CAD build for the part. Positions are in the model's coordinates, mm. A direction names the side the tool comes from. Give positions to 0.01 mm unless a question says otherwise; leave off trailing zeros. Write each loop counter-clockwise with the first axis right and the second up, starting at its lowest first coordinate (ties: lowest second). Pieces come first, ordered by that corner, then holes. Notation, with made-up numbers: (42, 70.25) - (92, 70.25) arc R30 ccw to (92, 105.25) - close; hole circle Ø11 at (2, -8.5). An arc over 180 degrees is marked (long way). Answer as a JSON object with one key per item and string values.
from build123d import *

# Parameters (mm, degrees)
CUT_EXTRUDE1_START = -4.25
SKETCH2_R          = 11.5
SKETCH2_R_2        = 11
CUT_EXTRUDE1_DEPTH = 1
CUT_EXTRUDE2_START = -12.75
SKETCH2_2_R        = 11.5
SKETCH2_2_R_2      = 11
CUT_EXTRUDE2_DEPTH = 1
SCALE1_SCALE       = 1.013


with BuildPart() as part:
    # Sketch1 → Revolve1 (revolve)
    with BuildSketch(Plane(origin=(0, 0, 0), x_dir=(0, 0, -1), z_dir=(1, 0, 0)), mode=Mode.PRIVATE) as revolve1_sk:
        with BuildLine():
            Line((-7, 11), (7, 11))
            Line((7, 11), (8, 12))
            Line((8, 12), (8, 19))
            ThreePointArc((8, 19), (7.707106781, 19.707106781), (7, 20))
            Line((7, 20), (6.5, 20))
            ThreePointArc((6.5, 20), (0, 13.5), (-6.5, 20))
            Line((-6.5, 20), (-7, 20))
            ThreePointArc((-7, 20), (-7.707106781, 19.707106781), (-8, 19))
            Line((-8, 19), (-8, 12))
            Line((-8, 12), (-7, 11))
        make_face()
    revolve(revolve1_sk.sketch.rotate(Axis((0, 0, 0), (0, 0, -1)), 90), axis=Axis((0, 0, 0), (0, 0, -1)))

    # Sketch2 → Cut-Extrude1 (cut)
    with BuildSketch(Plane.XY.offset(8).offset(CUT_EXTRUDE1_START)):
        Circle(SKETCH2_R)
        Circle(SKETCH2_R_2, mode=Mode.SUBTRACT)
    extrude(amount=CUT_EXTRUDE1_DEPTH, mode=Mode.SUBTRACT)

    # Sketch2_2 → Cut-Extrude2 (cut)
    with BuildSketch(Plane.XY.offset(8).offset(CUT_EXTRUDE2_START)):
        Circle(SKETCH2_2_R)
        Circle(SKETCH2_2_R_2, mode=Mode.SUBTRACT)
    extrude(amount=CUT_EXTRUDE2_DEPTH, mode=Mode.SUBTRACT)


with BuildPart() as part_1:
    # Scale1: scaled about (0, 0, 0)
    add(part.part.scale(SCALE1_SCALE))


solid = part_1.part
(1) Saw through at A-A, the plane z = 0.5. Give the cut face in (x, y).
Answer key:
{"outline": "circle Ø27.39 at (0, 0); hole circle Ø22.29 at (0, 0)"}
(2) Flat gauge pins, fed straight in: P1, Ø11.5, axis at x = -1.5, y = 2.5, coming from the -Z side; P2, Ø8, axis at x = 13, y = -16, coming from the +Z side; P3, Ø4, axis at x = -1, z = 1.5, coming from the -Y side; P4, Ø6, axis at x = 13, z = -1.5, coming from the +Y side. Where does each tip first touch, or does it go through?
Answer key:
{"P1": "passes through", "P2": "stops at z = 8.1", "P3": "stops at y = -14.65", "P4": "stops at y = 9.99"}
(3) Pull direction Z, two halves, no side cores. Call faces 1 (the face through (10.4, 4.3, -7.2)), 2 (the face through (11.11, 3.5, 4.3)), 3 (the face through (19.324, -6.086, -6.834)): pulls with the +Z half, pulls with the -Z half, needs draft (parallel to the pull), parting line crosses it, or undercut.
Answer key:
{"face 1": "pulls with the -Z half", "face 2": "undercut", "face 3": "needs draft"}
(4) 3-axis set-ups, long thin cutter, end or side, ignore diameter. For faces 4 (the face through (11.11, 3.5, -4.31)), 5 (the face through (10.628, -3.347, 5.935)): which of +Z, -Z, +X, -X, +Y, -Y reach the whole face in a straight line?
Answer key:
{"face 4": "none", "face 5": "+Z, -Z"}
(5) Probe L1, parallel to Z at x = 11.5, y = 1.5; L2, parallel to Y at x = 0, z = 1; L3, parallel to Y at x = -1.5, z = 2.25. List the from-to ranges inside material, lowest first. Write a range as [from, to].
Answer key:
{"L1": "z = [-7.55, -4.81], [-3.8, 3.8], [4.81, 7.55]", "L2": "y = [-13.75, -11.14], [11.14, 13.75]", "L3": "y = [-13.99, -11.04], [11.04, 13.99]"}
